from build123d import *

# Parameters (mm, degrees)
F2_W     = 780.327082
F2_H     = 355.154276
F3_DEPTH = 381


with BuildPart() as f1:
    # F0 (on Front) → F1 (revolve)
    with BuildSketch(Plane.XZ):
        Polygon((173.410069, 172.037573), (-80.589931, 172.037573), (-80.589931, -81.962427), align=None)
    revolve(axis=Axis((-80.589931, 0, 45.037573), (0, 0, -1)))

    # F2 (on Front) → F3 (join)
    with BuildSketch(Plane.XZ):
        with Locations((-33.309847, 40.15027)):
            Rectangle(F2_W, F2_H)
    extrude(amount=F3_DEPTH)


solid = f1.part
Here's how the part is built. I have some questions about the finished solid (model axes, mm). A direction names the side the tool comes from. Round coordinates to 2 decimals unless told otherwise and drop trailing zeros. Loops run counter-clockwise (first coordinate to the right, second up) from the corner with the lowest first, then second, coordinate; pieces in that order, holes last. Notation, with made-up numbers: (57, 52.5) - (90, 52.5) arc R13 ccw to (90, 56.5) - close; hole circle Ø8 at (14, 1.25). An arc over 180 degrees is marked (long way). One line per question, with ' | ' between items. Start each with the question number.
Q1. I want a section at B-B (z = -21). Write out the boundary of the cut face in (x, y), then the cut area to 3 significant figures.
Q2. I want a section at A-A (z = 94.5). Write out the boundary of the cut face in (x, y).
Q3. Will these pins go through, and if not, where does the flat tip stop? pin 1 (2 mm diameter, centred on x = 105, z = 178, fed in from +Y); pin 2 (4 mm diameter, centred on x = -127, z = 58, fed in from +Y).
Q4. For faces 1 (the flat face through (-84, 97, 172.038)), 2 (the flat face through (-423.473, -188, 38)), which set-ups out of +Z, -Z, +X, -X, +Y, -Y let a thin tool reach every point of the face, with its end or its side?
Q5. Please list where these lines run through material, in increasing order: line 1 (Y direction, x = 193.5, z = -108); line 2 (Z direction, x = -21, y = 195); line 3 (X direction, y = 58.5, z = 100). Write a range as [from, to].
Response values:
1) outline: (-423.47, -381) - (356.85, -381) - (356.85, 0) - (-19.63, 0) arc R60.96 ccw to (-141.55, 0) - (-423.47, 0) - close | area: 303,000 mm²
2) outline: (-423.47, -381) - (356.85, -381) - (356.85, 0) - (95.87, 0) arc R176.46 ccw to (-257.05, 0) - (-423.47, 0) - close
3) pin 1: stops at y = 0 | pin 2: stops at y = 134.27
4) face 1: +Z, +X, -X, +Y | face 2: +Z, -Z, -X, +Y, -Y
5) line 1: y = [-381, 0] | line 2: z = [121.94, 172.04] | line 3: x = [-252.89, 91.71]
